Geometry: final body of the model. Coordinates: model frame, mm. A direction names the side the tool comes from. Give positions to 0.01 mm unless a question says otherwise; leave off trailing zeros. Write each loop counter-clockwise with the first axis right and the second up, starting at its lowest first coordinate (ties: lowest second). Pieces come first, ordered by that corner, then holes. Notation, with made-up numbers: (-37.5, 76.5) -> (-11.5, 76.5) arc R34 ccw to (-11.5, 106.5) -> close; hole circle Ø3 at (-32.5, 52.25). An arc over 180 degrees is marked (long way). Answer as a JSON object with one key per item and string values. Group by question number.
(1) Draft query along X for faces 4 (the face through (15.875, -64, 0)), 5 (the face through (0, -66, 12.7)), 6 (the face through (-14.31, -95.66, 0.42)). Return one class per face: +X half, -X half, draft (parallel to the pull), parting line (faces both ways), or undercut.
(2) Material intervals for probe 1 along Z at (x, y) = (-8, -60.5) (3 decimals); probe 2 along Y at (x, z) = (-13.5, 2), sorted ascending.
(3) Section query C-C on x = -1.5. Output: boundary loops of the cut face in (y, z) (3 decimals).
(4) Set-up query: faces 1 (the face through (0, -72, -12.7)), 2 (the face through (0, -3.175, 11)), 3 (the face through (12.7, -66, 0)). Return all of +Z, -Z, +X, -X, +Y, -Y with unobstructed straight access to the full face (end or side cutting, diameter ignored); none if empty.
(5) Section query D-D on x = -14. Output: boundary loops of the cut face in (y, z) (3 decimals).
(6) Section query A-A on z = 0. Output: boundary loops of the cut face in (x, y) (3 decimals), plus the area to 3 significant figures.
(7) Section query B-B on y = -68. Output: boundary loops of the cut face in (x, z) (3 decimals), plus the area to 3 significant figures.
(8) Contact query for a flat-ended pin moving along its axis: pin 1 Ø1.5 at (x, z) = (-3.5, 11) entering from -Y (3 decimals). Output: stop coordinate, or through.
from build123d import *

# Parameters (mm, degrees)
F0_W     = 31.75
F0_H     = 31.75
F1_DEPTH = 130.599993
F2_T     = -3.175
F4_DEPTH = 50.8
F5_D     = 19.1008


with BuildPart() as f1:
    # F0 (on Front) → F1 (new body)
    with BuildSketch(Plane.XZ):
        Rectangle(F0_W, F0_H)
    extrude(amount=F1_DEPTH)

    # F2
    f2_openings = [f1.faces().sort_by_distance(p)[0] for p in [
        (0, -130.599993, 0),
    ]]
    offset(amount=F2_T, openings=f2_openings)

    # F3 (on face) → F4 (cut)
    with BuildSketch(Plane.YZ.offset(15.875)):
        Polygon((0, -15.875), (0, 15.875), (-16.299993, -15.875), align=None)
    extrude(amount=-F4_DEPTH, mode=Mode.SUBTRACT)

    # F5 (through all)
    with Locations(Plane.YZ.offset(15.875)):
        with Locations((-105.199993, 0)):
            Hole(F5_D / 2)


solid = f1.part
Answer list:
{
 "1": {"face 4": "+X half", "face 5": "undercut", "face 6": "draft"},
 "2": {"probe 1": "-15.875 to -12.7, 12.7 to 15.875", "probe 2": "-130.6 to -114.54, -95.86 to -7.12"},
 "3": {"outline": "(-130.6, -15.875) -> (-16.3, -15.875) -> (-14.67, -12.7) -> (-130.6, -12.7) -> close; (-130.6, 12.7) -> (-3.175, 12.7) -> (-3.175, 9.691) -> (0, 15.875) -> (-130.6, 15.875) -> close"},
 "4": {"face 1": "+Y, -Y", "face 2": "-Z, -Y", "face 3": "-Y"},
 "5": {"outline": "(-130.6, -15.875) -> (-16.3, -15.875) -> (0, 15.875) -> (-130.6, 15.875) -> close; hole circle Ø19.101 at (-105.2, 0)"},
 "6": {"outline": "(-15.875, -130.6) -> (-12.7, -130.6) -> (-12.7, -114.75) -> (-15.875, -114.75) -> close; (-15.875, -95.65) -> (-12.7, -95.65) -> (-12.7, -8.15) -> (-15.875, -8.15) -> close; (12.7, -130.6) -> (15.875, -130.6) -> (15.875, -114.75) -> (12.7, -114.75) -> close; (12.7, -95.65) -> (15.875, -95.65) -> (15.875, -8.15) -> (12.7, -8.15) -> close", "area": "656 mm2"},
 "7": {"outline": "(-15.875, -15.875) -> (15.875, -15.875) -> (15.875, 15.875) -> (-15.875, 15.875) -> close; hole (-12.7, -12.7) -> (12.7, -12.7) -> (12.7, 12.7) -> (-12.7, 12.7) -> close", "area": "363 mm2"},
 "8": {"pin 1": "y = -3.175"}
}
